Part model, mm, in its own coordinate system. A direction names the side the tool comes from. Round coordinates to 2 decimals unless told otherwise and drop trailing zeros. Write each loop counter-clockwise with the first axis right and the second up, starting at its lowest first coordinate (ties: lowest second). Pieces come first, ordered by that corner, then holes.
```python
from build123d import *

# Parameters (mm, degrees)
EXTRUDE_1_DEPTH          = 30
SKETCH_2_R               = 2.6
CUT_EXTRUDE_1_DEPTH      = 55.558317423
CUT_EXTRUDE_2_DEPTH      = 50.244289009
CUT_EXTRUDE_2_DEPTH_BACK = 50.244289009
SKETCH_3_R               = 1.5
SKETCH_4_W               = 10
SKETCH_4_H               = 6
CUT_EXTRUDE_3_DEPTH      = 55.558317423
EXTRUDE_START            = 6
SKETCH_5_R               = 2.65
SKETCH_5_R_2             = 1.5
EXTRUDE_2_DEPTH          = 6


with BuildPart() as part:
    # 草图1 → 凸台-拉伸1 (new body)
    with BuildSketch(Plane.XY):
        Polygon((-25, -5), (-13.1, -5), (-13.1, -25), (-10.1, -25), (-10.1, -5), (10.1, -5), (10.1, -25), (13.1, -25), (13.1, -5), (25, -5), (25, 5), (-25, 5), align=None)
    extrude(amount=EXTRUDE_1_DEPTH)

    # 草图2 → 切除-拉伸1 (cut, through all)
    with BuildSketch(Plane(origin=(13.1, 0, 0), x_dir=(0, 0, -1), z_dir=(1, 0, 0))):
        with Locations((-23, -15)):
            Circle(SKETCH_2_R)
        with Locations((-7, -15)):
            Circle(SKETCH_2_R)
    extrude(amount=-CUT_EXTRUDE_1_DEPTH, mode=Mode.SUBTRACT)

    # 草图3 → 切除-拉伸2 (cut, two sides: drawn at the far end of the back side and taken through both)
    with BuildSketch(Plane(origin=(0, 5, 0), x_dir=(1, 0, 0), z_dir=(0, 1, 0)).offset(-CUT_EXTRUDE_2_DEPTH_BACK)):
        with Locations(Location((16, -15, 0), (0, 0, 270))):
            Circle(SKETCH_3_R)
        with Locations(Location((-16, -15, 0), (0, 0, 180))):
            Circle(SKETCH_3_R)
    extrude(amount=CUT_EXTRUDE_2_DEPTH + CUT_EXTRUDE_2_DEPTH_BACK, mode=Mode.SUBTRACT)

    # 草图4 → 切除-拉伸3 (cut, through all)
    with BuildSketch(Plane(origin=(13.1, 0, 0), x_dir=(0, 0, -1), z_dir=(1, 0, 0))):
        with Locations((-15, -8)):
            Rectangle(SKETCH_4_W, SKETCH_4_H)
    extrude(amount=-CUT_EXTRUDE_3_DEPTH, mode=Mode.SUBTRACT)

    # 草图5 → 凸台-拉伸2 (add)
    # profile 1 of 2: a face of its own
    with BuildSketch(Plane(origin=(0, 5, 0), x_dir=(1, 0, 0), z_dir=(0, 1, 0)).offset(EXTRUDE_START)):
        with Locations((16, -15)):
            Circle(SKETCH_5_R)
        with Locations(Location((16, -15, 0), (0, 0, 180))):
            Circle(SKETCH_5_R_2, mode=Mode.SUBTRACT)
    # profile 2 of 2: a face of its own
    with BuildSketch(Plane(origin=(0, 5, 0), x_dir=(1, 0, 0), z_dir=(0, 1, 0)).offset(EXTRUDE_START)):
        with Locations((-16, -15)):
            Circle(SKETCH_5_R)
        with Locations(Location((-16, -15, 0), (0, 0, 180))):
            Circle(SKETCH_5_R_2, mode=Mode.SUBTRACT)
    extrude(amount=-EXTRUDE_2_DEPTH)


solid = part.part
```
Q1. Cut at D-D on z = 15. Write the cut outline in (x, y), plus the area to 3 significant figures.
Values follow:
outline: (-25, -5) - (-17.5, -5) - (-17.5, 11) - (-18.65, 11) - (-18.65, 5) - (-25, 5) - close; (-14.5, -5) - (14.5, -5) - (14.5, 11) - (13.35, 11) - (13.35, 5) - (-13.35, 5) - (-13.35, 11) - (-14.5, 11) - close; (-13.1, -25) - (-10.1, -25) - (-10.1, -11) - (-13.1, -11) - close; (10.1, -25) - (13.1, -25) - (13.1, -11) - (10.1, -11) - close; (17.5, -5) - (25, -5) - (25, 5) - (18.65, 5) - (18.65, 11) - (17.5, 11) - close
area: 552 mm2
Q2. Which spindle directions (+Z, -Z, +X, -X, +Y, -Y) get a long thin tool onto all of the face, cutting with end or side? Do faces 1 (the flat face through (12, -8, 10)), 2 (the flat face through (-25, 0, 15)), 3 (the flat face through (-13.1, -15, 15)), 4 (the flat face through (13.1, -15, 15)), 5 (the cylindrical face through (-13.55, 8.04, 16.01)). Say none if no direction does.
Values follow:
face 1: +X, -X
face 2: +Z, -Z, -X, +Y, -Y
face 3: +Z, -Z, -X, -Y
face 4: +Z, -Z, +X, -Y
face 5: +Y
Q3. Cut at A-A on z = 6. Write the cut outline in (x, y), plus the area to 3 significant figures.
Values follow:
outline: (-25, -5) - (-13.1, -5) - (-13.1, -12.6) - (-10.1, -12.6) - (-10.1, -5) - (10.1, -5) - (10.1, -12.6) - (13.1, -12.6) - (13.1, -5) - (25, -5) - (25, 5) - (-25, 5) - close; (-13.1, -25) - (-10.1, -25) - (-10.1, -17.4) - (-13.1, -17.4) - close; (10.1, -25) - (13.1, -25) - (13.1, -17.4) - (10.1, -17.4) - close
area: 591 mm2
Q4. Cut at C-C on x = 16. Write the cut outline in (y, z).
Values follow:
outline: (-5, 0) - (5, 0) - (5, 12.35) - (11, 12.35) - (11, 13.5) - (-5, 13.5) - close; (-5, 16.5) - (11, 16.5) - (11, 17.65) - (5, 17.65) - (5, 30) - (-5, 30) - close
Q5. Drop flat-ended pins along their axis: pin 1 (6 mm diameter, centred on y = -17.5, z = 10.5, fed in from -X); pin 2 (2.5 mm diameter, centred on x = -16, z = 15, fed in from -Y); pin 3 (1 mm diameter, centred on x = -18.5, z = 15, fed in from -Y); pin 4 (6 mm diameter, centred on y = -15, z = 23, fed in from +X). Give the stop position or say it passes through.
Values follow:
pin 1: stops at x = -13.1
pin 2: passes through
pin 3: stops at y = -5
pin 4: stops at x = 13.1
Q6. Cut at B-B on y = -15. Write the cut outline in (x, z), plus the area to 3 significant figures.
Values follow:
outline: (-13.1, 0) - (-10.1, 0) - (-10.1, 4.4) - (-13.1, 4.4) - close; (-13.1, 9.6) - (-10.1, 9.6) - (-10.1, 20.4) - (-13.1, 20.4) - close; (-13.1, 25.6) - (-10.1, 25.6) - (-10.1, 30) - (-13.1, 30) - close; (10.1, 0) - (13.1, 0) - (13.1, 4.4) - (10.1, 4.4) - close; (10.1, 9.6) - (13.1, 9.6) - (13.1, 20.4) - (10.1, 20.4) - close; (10.1, 25.6) - (13.1, 25.6) - (13.1, 30) - (10.1, 30) - close
area: 118 mm2
Q7. Mould opens along Z. For faces 6 (the flat face through (12, -25, 15)), 7 (the flat face through (12, -11, 15)), 8 (the flat face through (0, -3, 30)) say: +Z half, -Z half, draft (parallel to the pull), parting line (faces both ways), or undercut.
Values follow:
face 6: draft
face 7: undercut
face 8: +Z half
Q8. Wall check: L1, parallel to X at y = 9.2, z = 15; L2, parallel to Y at x = 12.45, z = 7; L3, parallel to Z at x = 16, y = 7. Give the ranges that are in metal, low to high.
Values follow:
L1: x = -18.65 to -17.5, -14.5 to -13.35, 13.35 to 14.5, 17.5 to 18.65
L2: y = -25 to -17.6, -12.4 to 5
L3: z = 12.35 to 13.5, 16.5 to 17.65
